```python
from build123d import *

# Parameters (mm, degrees)
F0_W     = 57.15
F0_H     = 44.45
F1_DEPTH = 25.4
F3_DEPTH = 12.7
F5_DEPTH = 25.401
F7_DEPTH = 25.4


with BuildPart() as f1:
    # F0 (on Front) → F1 (new body)
    with BuildSketch(Plane.XZ):
        with Locations((-26.4685656875, 7.2840715903)):
            Rectangle(F0_W, F0_H)
    extrude(amount=F1_DEPTH)

    # F2 (on face) → F3 (cut)
    with BuildSketch(Plane.XZ.offset(25.4)):
        Polygon((2.1064343125, 29.5090715903), (-40.8858768642, 29.5090715903), (-8.9903669432, -14.9409284097), (2.1064343125, -14.9409284097), align=None)
    extrude(amount=-F3_DEPTH, mode=Mode.SUBTRACT)

    # F4 (on face) → F5 (cut, through all)
    with BuildSketch(Plane.XZ.offset(25.4)):
        with BuildLine():
            Line((-19.7113687501, 0), (-34.6783755455, 20.8582165233))
            ThreePointArc((-34.6783755455, 20.8582165233), (-37.7301963147, 2.8693886556), (-19.7113687501, 0))
        make_face()
    extrude(amount=-F5_DEPTH, mode=Mode.SUBTRACT)

    # F6 (on face) → F7 (cut)
    with BuildSketch(Plane.XZ.offset(12.7)):
        with BuildLine():
            Line((-34.6783755455, 20.8582165233), (-19.7113687501, 0))
            ThreePointArc((-19.7113687501, 0), (-16.6145780918, 18.0210964288), (-34.6783755455, 20.8582165233))
        make_face()
    extrude(amount=-F7_DEPTH, mode=Mode.SUBTRACT)


solid = f1.part
```
For this review, take the finished solid that the model builds, in its own axes (mm). A direction names the side the tool comes from. Round coordinates to 2 decimals unless told otherwise and drop trailing zeros. Loops run counter-clockwise (first coordinate to the right, second up) from the corner with the lowest first, then second, coordinate; pieces in that order, holes last.
Q1. Add section B-B on x = -23. Write out the cut boundary in (y, z), plus the area to 3 significant figures.
Result sheet:
outline: (-25.4, -14.94) - (0, -14.94) - (0, -1.74) - (-25.4, -1.74) - close; (-12.7, 22.72) - (0, 22.72) - (0, 29.51) - (-12.7, 29.51) - close
area: 421 mm2
Q2. Machinability: for faces 5 (the face through (-37.826, -19.139, 25.244)), 6 (the face through (-21, 0, -2)), which of the approach directions +Z, -Z, +X, -X, +Y, -Y give a long, thin tool a straight path to every point of the face, cutting with its end or side? Answer none if there is none.
Result sheet:
face 5: +Z, +X, -Y
face 6: +Z, -Z, +X, -X, +Y
Q3. Add section C-C on y = -3. Write out the cut boundary in (x, z).
Result sheet:
outline: (-55.04, -14.94) - (2.11, -14.94) - (2.11, 29.51) - (-55.04, 29.51) - close; hole (-34.68, 20.86) arc R12.84 ccw (long way) to (-19.71, 0) arc R12.84 ccw (long way) to start
Q4. Add section D-D on y = -15. Write out the cut boundary in (x, z).
Result sheet:
outline: (-55.04, -14.94) - (-8.99, -14.94) - (-19.71, 0) arc R12.84 cw (long way) to (-34.68, 20.86) - (-40.89, 29.51) - (-55.04, 29.51) - close
Q5. Add section A-A on z = 13. Write out the cut boundary in (x, y).
Result sheet:
outline: (-55.04, -25.4) - (-39.86, -25.4) - (-39.86, 0) - (-55.04, 0) - close; (-14.45, -12.7) - (2.11, -12.7) - (2.11, 0) - (-14.45, 0) - close
Q6. Mouldability with a two-part tool opening along X and no side actions: class faces 1 (the face through (-14.4, -19.1, -7.4)), 2 (the face through (-37.89, -12.88, 3.1)), 3 (the face through (-33, -10, 29.509)), 4 (the face through (-55.044, -13, 7)) as +X half, -X half, draft (parallel to the pull), parting line (faces both ways), or undercut.
Result sheet:
face 1: +X half
face 2: undercut
face 3: draft
face 4: -X half
Q7. Insertion check: pin 1 Ø12 at (x, z) = (-25, 15) entering from +Y; pin 2 Ø21.5 at (x, z) = (-20, 12) entering from -Y. Each pin has a flat end and moves straight along its axis. Give the tip position at first contact, or say it passes through.
Result sheet:
pin 1: passes through
pin 2: stops at y = -12.7
Q8. To check wall thickness, follow line 1 along Z through (x, y) = (-22, -4); line 2 along Y through (x, z) = (-36, 26.5); line 3 along Z through (x, y) = (-16, -5.5). State the ranges of each line that lie inside material, in increasing order.
Result sheet:
line 1: z = -14.94 to -1.34, 22.34 to 29.51
line 2: y = -12.7 to 0
line 3: z = -14.94 to 3.99, 17.08 to 29.51
